Model file for the job. Use its own axes, mm. A direction names the side the tool comes from. Round coordinates to 2 decimals unless told otherwise and drop trailing zeros. Loops run counter-clockwise (first coordinate to the right, second up) from the corner with the lowest first, then second, coordinate; pieces in that order, holes last. Notation, with made-up numbers: (-5.5, 86) - (8.5, 86) arc R18 ccw to (8.5, 96) - close; hole circle Ø6 at (-4, -16). An arc over 180 degrees is marked (long way). Use one line per item in the form item = value.
from build123d import *

# Parameters (mm, degrees)
SKETCH1_W               = 100
SKETCH1_H               = 26
BOSS_EXTRUDE1_DEPTH     = 2
BOSS_EXTRUDE2_DEPTH     = 100
SKETCH3_W               = 25
SKETCH3_H               = 28
BOSS_EXTRUDE3_DEPTH     = 4
SKETCH4_R               = 2.1
CUT_EXTRUDE1_DEPTH      = 106.39449701
SKETCH5_W               = 120
SKETCH5_H               = 46
SKETCH5_W_2             = 100
SKETCH5_H_2             = 26
CUT_EXTRUDE2_DEPTH      = 105.537074763
CUT_EXTRUDE2_DEPTH_BACK = 105.537074763
SKETCH6_W               = 100
SKETCH6_H               = 26
SKETCH6_R               = 3.6
BOSS_EXTRUDE4_DEPTH     = 4.2
SKETCH8_W               = 100
SKETCH8_H               = 4
BOSS_EXTRUDE5_DEPTH     = 6
SKETCH9_W               = 100
SKETCH9_H               = 4
BOSS_EXTRUDE6_DEPTH     = 10.2
SKETCH10_W              = 4
SKETCH10_H              = 37.5
CUT_EXTRUDE3_DEPTH      = 106.682732743
SKETCH11_W              = 4
SKETCH11_H              = 25
CUT_EXTRUDE4_DEPTH      = 107.737247482
SKETCH13_W              = 10
SKETCH13_H              = 10
BOSS_EXTRUDE7_DEPTH     = 6.2
SKETCH14_W              = 4.2
SKETCH14_H              = 35.5
CUT_EXTRUDE5_DEPTH      = 107.737247482
SKETCH15_R              = 3.6
BOSS_EXTRUDE8_DEPTH     = 6
SKETCH17_R              = 1.75
CUT_EXTRUDE7_DEPTH      = 105.984951303
MOVE_FACE2_BY           = 2


with BuildPart() as part:
    # Sketch1 → Boss-Extrude1 (new body)
    with BuildSketch(Plane(origin=(0, 0, 0), x_dir=(0, 0, -1), z_dir=(1, 0, 0))):
        with Locations((50, 13)):
            Rectangle(SKETCH1_W, SKETCH1_H)
    extrude(amount=BOSS_EXTRUDE1_DEPTH)

    # Sketch2 → Boss-Extrude2 (add)
    with BuildSketch(Plane.XY):
        Polygon((2, 26), (2, 28), (-12, 28), (-12, 24), (-10, 24), (-10, 26), align=None)
    extrude(amount=-BOSS_EXTRUDE2_DEPTH)

    # Sketch3 → Boss-Extrude3 (add)
    with BuildSketch(Plane(origin=(2, 0, 0), x_dir=(0, 0, -1), z_dir=(1, 0, 0))):
        with Locations((50, 14)):
            Rectangle(SKETCH3_W, SKETCH3_H)
    extrude(amount=BOSS_EXTRUDE3_DEPTH)

    # Sketch4 → Cut-Extrude1 (cut, through all)
    with BuildSketch(Plane(origin=(6, 0, 0), x_dir=(0, 0, -1), z_dir=(1, 0, 0))):
        with Locations((41.5, 21)):
            Circle(SKETCH4_R)
        with Locations((58.5, 21)):
            Circle(SKETCH4_R)
        with Locations((58.5, 4)):
            Circle(SKETCH4_R)
        with Locations((41.5, 4)):
            Circle(SKETCH4_R)
    extrude(amount=-CUT_EXTRUDE1_DEPTH, mode=Mode.SUBTRACT)


with BuildPart() as body_2:
    # Mirror1: mirrored copy
    add(part.part.mirror(Plane(origin=(6, 0, 0), x_dir=(0, 0, 1), z_dir=(1, 0, 0))))

    # Sketch5 → Cut-Extrude2 (cut, two sides)
    with BuildSketch(Plane(origin=(12, 0, 0), x_dir=(0, 0, -1), z_dir=(1, 0, 0))) as cut_extrude2_sk:
        with Locations((50, 13)):
            Rectangle(SKETCH5_W, SKETCH5_H)
        with Locations((50, 13)):
            Rectangle(SKETCH5_W_2, SKETCH5_H_2, mode=Mode.SUBTRACT)
    extrude(amount=CUT_EXTRUDE2_DEPTH, mode=Mode.SUBTRACT)
    extrude(cut_extrude2_sk.sketch, amount=-CUT_EXTRUDE2_DEPTH_BACK, mode=Mode.SUBTRACT)


with BuildPart() as body_2_2:
    # of the pieces the cut leaves, the one that is kept (cut_extrude2_keep)
    add(body_2.part.solids().sort_by_distance((12, 0, 0))[0])

    # Sketch6 → Boss-Extrude4 (add)
    with BuildSketch(Plane(origin=(12, 0, 0), x_dir=(0, 0, -1), z_dir=(1, 0, 0))):
        with Locations((50, 13)):
            Rectangle(SKETCH6_W, SKETCH6_H)
        with Locations((41.5, 21)):
            Circle(SKETCH6_R, mode=Mode.SUBTRACT)
        with Locations((58.5, 21)):
            Circle(SKETCH6_R, mode=Mode.SUBTRACT)
        with Locations((58.5, 4)):
            Circle(SKETCH6_R, mode=Mode.SUBTRACT)
        with Locations((41.5, 4)):
            Circle(SKETCH6_R, mode=Mode.SUBTRACT)
    extrude(amount=BOSS_EXTRUDE4_DEPTH)



with BuildPart() as body_2_3:
    # Sketch8 → Boss-Extrude5 (new body)
    with BuildSketch(Plane(origin=(16.2, 0, 0), x_dir=(0, 0, -1), z_dir=(1, 0, 0))):
        with Locations((50, -2)):
            Rectangle(SKETCH8_W, SKETCH8_H)
    extrude(amount=BOSS_EXTRUDE5_DEPTH)


with BuildPart() as body_2_2_1:
    add(body_2_2.part)

    add(body_2_3.part)  # Boss-Extrude6 merges body 2 3
    # Sketch9 → Boss-Extrude6 (add)
    with BuildSketch(Plane.ZY.offset(-16.2)):
        with Locations((-50, -2)):
            Rectangle(SKETCH9_W, SKETCH9_H)
    extrude(amount=BOSS_EXTRUDE6_DEPTH)

    # Sketch10 → Cut-Extrude3 (cut, through all)
    with BuildSketch(Plane(origin=(0, 0, 0), x_dir=(1, 0, 0), z_dir=(0, 1, 0))):
        with Locations((8, 81.25)):
            Rectangle(SKETCH10_W, SKETCH10_H)
        with Locations((8, 18.75)):
            Rectangle(SKETCH10_W, SKETCH10_H)
    extrude(amount=-CUT_EXTRUDE3_DEPTH, mode=Mode.SUBTRACT)

    # Sketch11 → Cut-Extrude4 (cut, through all)
    with BuildSketch(Plane(origin=(0, 26, 0), x_dir=(1, 0, 0), z_dir=(0, 1, 0))):
        with Locations((8, 50)):
            Rectangle(SKETCH11_W, SKETCH11_H)
    extrude(amount=-CUT_EXTRUDE4_DEPTH, mode=Mode.SUBTRACT)

    # Sketch13 → Boss-Extrude7 (add)
    with BuildSketch(Plane.ZY.offset(-10)):
        with Locations((-50, 31)):
            Rectangle(SKETCH13_W, SKETCH13_H)
    extrude(amount=-BOSS_EXTRUDE7_DEPTH)

    # Sketch14 → Cut-Extrude5 (cut, through all)
    with BuildSketch(Plane(origin=(0, 26, 0), x_dir=(1, 0, 0), z_dir=(0, 1, 0))):
        with Locations((12.1, 17.75)):
            Rectangle(SKETCH14_W, SKETCH14_H)
        with Locations((12.1, 82.25)):
            Rectangle(SKETCH14_W, SKETCH14_H)
    extrude(amount=-CUT_EXTRUDE5_DEPTH, mode=Mode.SUBTRACT)

    # Sketch15 → Boss-Extrude8 (add)
    with BuildSketch(Plane(origin=(22.2, 0, 0), x_dir=(0, 0, -1), z_dir=(1, 0, 0))):
        Polygon((0, 0), (100, 0), (100, 13), (57.5, 13), (57.5, 11.5), (42.5, 11.5), (42.5, 13), (0, 13), align=None)
        with Locations((41.5, 4)):
            Circle(SKETCH15_R, mode=Mode.SUBTRACT)
        with Locations((58.5, 4)):
            Circle(SKETCH15_R, mode=Mode.SUBTRACT)
    extrude(amount=-BOSS_EXTRUDE8_DEPTH)

    # Sketch17 → Cut-Extrude7 (cut, through all)
    with BuildSketch(Plane(origin=(0, 13, 0), x_dir=(1, 0, 0), z_dir=(0, 1, 0))):
        with Locations(Location((19.2, 34.15, 0), (0, 0, 270))):
            Circle(SKETCH17_R)
        with Locations(Location((19.2, 66.71679058, 0), (0, 0, 270))):
            Circle(SKETCH17_R)
    extrude(amount=-CUT_EXTRUDE7_DEPTH, mode=Mode.SUBTRACT)

    # Move Face2: a face moved inward by 2.0
    extrude(body_2_2_1.faces().sort_by_distance((17.355486439, -4, -49.990760145))[0], amount=MOVE_FACE2_BY, dir=(0, 1, 0), mode=Mode.SUBTRACT)


solid = body_2_2_1.part
1. Cut at A-A, the plane y = 4. Give the cut face in (x, z).
Geometry check:
outline = (10, -64.5) - (14.2, -64.5) - (14.2, -100) - (22.2, -100) - (22.2, -62.1) - (12, -62.1) - (12, -60.6) - (10, -60.6) - close; (10, -56.4) - (12, -56.4) - (12, -54.9) - (22.2, -54.9) - (22.2, -45.1) - (12, -45.1) - (12, -43.6) - (10, -43.6) - close; (10, -39.4) - (12, -39.4) - (12, -37.9) - (22.2, -37.9) - (22.2, 0) - (14.2, 0) - (14.2, -35.5) - (10, -35.5) - close; hole circle Ø3.5 at (19.2, -66.72); hole circle Ø3.5 at (19.2, -34.15)
2. Wall check: probe 1 along Z at (x, y) = (10.95, 4); probe 2 along Y at (x, z) = (11.25, -41.5); probe 3 along Z at (x, y) = (18, 0). Give the ranges that are in metal, low to high.
Geometry check:
probe_1 = -64.5 to -60.6, -56.4 to -43.6, -39.4 to -35.5
probe_2 = -2 to 1.9, 6.1 to 18.9, 23.1 to 26
probe_3 = -100 to -67.99, -65.44 to -35.42, -32.88 to 0
3. Cut at B-B, the plane z = -34.15. Give the cut face in (x, y).
Geometry check:
outline = (14.2, -2) - (17.45, -2) - (17.45, 13) - (16.2, 13) - (16.2, 26) - (14.2, 26) - close; (20.95, -2) - (22.2, -2) - (22.2, 13) - (20.95, 13) - close
4. Flat gauge pins, fed straight in: pin 1 (7 mm diameter, centred on x = 13.5, z = -13.5, fed in from +Y); pin 2 (3 mm diameter, centred on y = 23.5, z = -25.5, fed in from -X); pin 3 (5.5 mm diameter, centred on y = 4, z = -58.5, fed in from +X). Where does each tip first touch, or does it go through?
Geometry check:
pin_1 = 26
pin_2 = 14.2
pin_3 = 12
5. Cut at D-D, the plane z = -58.5. Give the cut face in (x, y), plus the area to 3 significant figures.
Geometry check:
outline = (10, -2) - (22.2, -2) - (22.2, 0.4) - (12, 0.4) - (12, 1.9) - (10, 1.9) - close; (10, 6.1) - (12, 6.1) - (12, 7.6) - (22.2, 7.6) - (22.2, 13) - (16.2, 13) - (16.2, 17.4) - (12, 17.4) - (12, 18.9) - (10, 18.9) - close; (10, 23.1) - (12, 23.1) - (12, 24.6) - (16.2, 24.6) - (16.2, 26) - (10, 26) - close
area = 143 mm^2
6. Cut at C-C, the plane x = 19.2. Give the cut face in (y, z).
Geometry check:
outline = (-2, -100) - (13, -100) - (13, -68.47) - (-2, -68.47) - close; (-2, -64.97) - (13, -64.97) - (13, -57.5) - (11.5, -57.5) - (11.5, -42.5) - (13, -42.5) - (13, -35.9) - (-2, -35.9) - close; (-2, -32.4) - (13, -32.4) - (13, 0) - (-2, 0) - close; hole circle Ø7.2 at (4, -58.5); hole circle Ø7.2 at (4, -41.5)
7. Pull direction Y, two halves, no side cores. Call faces 5 (the flat face through (19, 13, -22)), 6 (the flat face through (10, 13, -50)), 7 (the flat face through (12, 2, -43)): +Y half, -Y half, draft (parallel to the pull), parting line (faces both ways), or undercut.
Geometry check:
face_5 = +Y half
face_6 = draft
face_7 = undercut
8. Tool access for faces 1 (the flat face through (12, 12, -64.5)), 2 (the flat face through (19, 13, -79)), 3 (the flat face through (12, 2, -60)), 4 (the flat face through (13, 31, -55)): list every direction of +Z, -Z, +X, -X, +Y, -Y with a clear straight run to the whole face (end or side of a thin tool).
Geometry check:
face_1 = -Z, -X, +Y, -Y
face_2 = +Z, -Z, +X, +Y
face_3 = +X
face_4 = -Z, +X, -X, +Y
